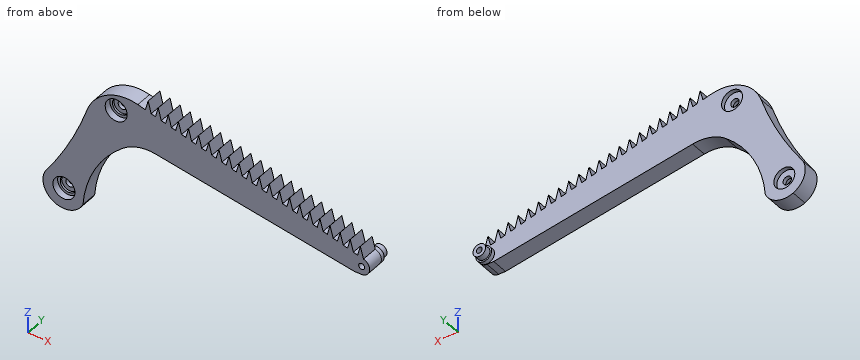
from build123d import *

# Parameters (mm, degrees)
SKETCH1_R                = 1.4
BOSS_EXTRUDE1_DEPTH      = 8
SKETCH2_R                = 3.75
BOSS_EXTRUDE2_DEPTH      = 2
SKETCH3_R                = 3
BOSS_EXTRUDE3_DEPTH      = 3
CUT_EXTRUDE1_DEPTH       = 153.777621068
CUT_EXTRUDE1_DEPTH_BACK  = 153.777621068
SKETCH4_R                = 1.4
FILLET1_R                = 4
SKETCH5_R                = 5.1
CUT_EXTRUDE2_DEPTH       = 3.2
SKETCH6_R                = 4
CUT_EXTRUDE3_DEPTH       = 1
SKETCH7_R                = 5
CUT_EXTRUDE4_DEPTH       = 2
CUT_EXTRUDE5_DEPTH       = 128.709870942
CUT_EXTRUDE5_DEPTH_BACK  = 128.709870942
SKETCH8_R                = 2
SKETCH9_W                = 150
SKETCH9_H                = 50
CUT_EXTRUDE6_DEPTH       = 128.657240829
BOSS_EXTRUDE4_DEPTH      = 8
FILLET2_R                = 10
SKETCH11_R               = 5.25
CUT_EXTRUDE7_DEPTH       = 3.2
SKETCH12_R               = 4
CUT_EXTRUDE8_DEPTH       = 1
SKETCH13_R               = 5
CUT_EXTRUDE9_DEPTH       = 2
CUT_EXTRUDE10_DEPTH      = 128.709870942
CUT_EXTRUDE10_DEPTH_BACK = 128.709870942
SKETCH14_R               = 2
CUT_EXTRUDE11_DEPTH      = 128.657240829
CUT_EXTRUDE11_DEPTH_BACK = 128.657240829
FILLET3_R                = 20
CUT_EXTRUDE12_DEPTH      = 128.657240829
CUT_EXTRUDE12_DEPTH_BACK = 128.657240829
FILLET4_R                = 20
FILLET5_R                = 20
BOSS_EXTRUDE5_DEPTH      = 8
LPATTERN1_COUNT          = 22
LPATTERN1_PITCH          = 5
SKETCH19_R               = 5.25
CUT_EXTRUDE13_DEPTH      = 3.2
SKETCH20_R               = 4
CUT_EXTRUDE14_DEPTH      = 1
CUT_EXTRUDE15_DEPTH      = 129.03726605
CUT_EXTRUDE15_DEPTH_BACK = 129.03726605
SKETCH21_R               = 2
SKETCH22_R               = 5
CUT_EXTRUDE16_DEPTH      = 2


# Some blends are built 0.0001 mm under size
with BuildPart() as part:
    # Sketch1 → Boss-Extrude1 (new body)
    with BuildSketch(Plane(origin=(0, 0, 0), x_dir=(1, 0, 0), z_dir=(0, 1, 0))):
        Polygon((-146.874100845, 0), (146.874100845, 0), (0, -40), align=None)
        with Locations(Location((-117.130755004, -3.915785767, 0), (0, 0, 270))):
            Circle(SKETCH1_R, mode=Mode.SUBTRACT)
        with Locations(Location((0, -30, 0), (0, 0, 270))):
            Circle(SKETCH1_R, mode=Mode.SUBTRACT)
        with Locations(Location((117.130755004, -3.915785767, 0), (0, 0, 270))):
            Circle(SKETCH1_R, mode=Mode.SUBTRACT)
    extrude(amount=BOSS_EXTRUDE1_DEPTH)

    # Sketch2 → Boss-Extrude2 (add)
    with BuildSketch(Plane(origin=(0, 8, 0), x_dir=(1, 0, 0), z_dir=(0, 1, 0))):
        with Locations(Location((117.130755004, -3.915785767, 0), (0, 0, 90))):
            Circle(SKETCH2_R)
    extrude(amount=BOSS_EXTRUDE2_DEPTH)

    # Sketch3 → Boss-Extrude3 (add)
    with BuildSketch(Plane(origin=(0, 10, 0), x_dir=(1, 0, 0), z_dir=(0, 1, 0))):
        with Locations(Location((117.130755004, -3.915785767, 0), (0, 0, 270))):
            Circle(SKETCH3_R)
    extrude(amount=BOSS_EXTRUDE3_DEPTH)

    # Sketch4 → Cut-Extrude1 (cut, two sides: drawn at the far end of the back side and taken through both)
    with BuildSketch(Plane(origin=(0, 13, 0), x_dir=(1, 0, 0), z_dir=(0, 1, 0)).offset(-CUT_EXTRUDE1_DEPTH_BACK)):
        with Locations(Location((117.130755004, -3.915785767, 0), (0, 0, 270))):
            Circle(SKETCH4_R)
    extrude(amount=CUT_EXTRUDE1_DEPTH + CUT_EXTRUDE1_DEPTH_BACK, mode=Mode.SUBTRACT)

    # Fillet1
    fillet1_edges = [part.edges().sort_by_distance(p)[0] for p in [
        (-146.874100845, 4, 0),
        (146.874100845, 4, 0),
    ]]
    fillet(fillet1_edges, radius=FILLET1_R)

    # Sketch5 → Cut-Extrude2 (cut)
    with BuildSketch(Plane.XZ):
        with Locations((-117.130755004, 3.915785767)):
            Circle(SKETCH5_R)
    extrude(amount=-CUT_EXTRUDE2_DEPTH, mode=Mode.SUBTRACT)

    # Sketch6 → Cut-Extrude3 (cut)
    with BuildSketch(Plane.XZ.offset(-3.2)):
        with Locations((-117.130755004, 3.915785767)):
            Circle(SKETCH6_R)
    extrude(amount=-CUT_EXTRUDE3_DEPTH, mode=Mode.SUBTRACT)

    # Sketch7 → Cut-Extrude4 (cut)
    with BuildSketch(Plane(origin=(0, 8, 0), x_dir=(1, 0, 0), z_dir=(0, 1, 0))):
        with Locations((-117.130755004, -3.915785767)):
            Circle(SKETCH7_R)
    extrude(amount=-CUT_EXTRUDE4_DEPTH, mode=Mode.SUBTRACT)

    # Sketch8 → Cut-Extrude5 (cut, two sides: drawn at the far end of the back side and taken through both)
    with BuildSketch(Plane.XZ.offset(-4.2).offset(-CUT_EXTRUDE5_DEPTH_BACK)):
        with Locations(Location((-117.130755004, 3.915785767, 0), (0, 0, 270))):
            Circle(SKETCH8_R)
    extrude(amount=CUT_EXTRUDE5_DEPTH + CUT_EXTRUDE5_DEPTH_BACK, mode=Mode.SUBTRACT)

    # Sketch9 → Cut-Extrude6 (cut, through all)
    with BuildSketch(Plane(origin=(0, 8, 0), x_dir=(1, 0, 0), z_dir=(0, 1, 0))):
        with Locations((-85, -25)):
            Rectangle(SKETCH9_W, SKETCH9_H)
    extrude(amount=-CUT_EXTRUDE6_DEPTH, mode=Mode.SUBTRACT)

    # Sketch10 → Boss-Extrude4 (add)
    with BuildSketch(Plane(origin=(0, 8, 0), x_dir=(1, 0, 0), z_dir=(0, 1, 0))):
        Polygon((-10, -37.276579072), (-38.232590814, 23.268407311), (-20.106435073, 31.720772546), (-5.314795912, 0), (-10, 0), align=None)
    extrude(amount=-BOSS_EXTRUDE4_DEPTH)

    # Fillet2
    fillet2_edges = [part.edges().sort_by_distance(p)[0] for p in [
        (-20.106435073, 4, -31.720772546),
        (-38.232590814, 4, -23.268407311),
    ]]
    fillet(fillet2_edges, radius=FILLET2_R - 0.0001)  # a hair under: the kernel refuses the full size

    # Sketch11 → Cut-Extrude7 (cut)
    with BuildSketch(Plane.XZ):
        with Locations(Location((-24.943330326, -18.431512059, 0), (0, 0, 270))):
            Circle(SKETCH11_R)
    extrude(amount=-CUT_EXTRUDE7_DEPTH, mode=Mode.SUBTRACT)

    # Sketch12 → Cut-Extrude8 (cut)
    with BuildSketch(Plane.XZ.offset(-3.2)):
        with Locations(Location((-24.943330326, -18.431512059, 0), (0, 0, 270))):
            Circle(SKETCH12_R)
    extrude(amount=-CUT_EXTRUDE8_DEPTH, mode=Mode.SUBTRACT)

    # Sketch13 → Cut-Extrude9 (cut)
    with BuildSketch(Plane(origin=(0, 8, 0), x_dir=(1, 0, 0), z_dir=(0, 1, 0))):
        with Locations(Location((-24.943330326, 18.431512059, 0), (0, 0, 270))):
            Circle(SKETCH13_R)
    extrude(amount=-CUT_EXTRUDE9_DEPTH, mode=Mode.SUBTRACT)

    # Sketch14 → Cut-Extrude10 (cut, two sides: drawn at the far end of the back side and taken through both)
    with BuildSketch(Plane.XZ.offset(-4.2).offset(-CUT_EXTRUDE10_DEPTH_BACK)):
        with Locations(Location((-24.943330326, -18.431512059, 0), (0, 0, 270))):
            Circle(SKETCH14_R)
    extrude(amount=CUT_EXTRUDE10_DEPTH + CUT_EXTRUDE10_DEPTH_BACK, mode=Mode.SUBTRACT)

    # Sketch16 → Cut-Extrude11 (cut, two sides: drawn at the far end of the back side and taken through both)
    with BuildSketch(Plane(origin=(0, 8, 0), x_dir=(1, 0, 0), z_dir=(0, 1, 0)).offset(-CUT_EXTRUDE11_DEPTH_BACK)):
        Polygon((-5.314795912, 0), (3.729692447, -19.395967878), (113.729692447, 0), align=None)
    extrude(amount=CUT_EXTRUDE11_DEPTH + CUT_EXTRUDE11_DEPTH_BACK, mode=Mode.SUBTRACT)

    # Fillet3
    fillet3_edges = [part.edges().sort_by_distance(p)[0] for p in [
        (3.729692447, 4, 19.395967878),
    ]]
    fillet(fillet3_edges, radius=FILLET3_R)

    # Sketch17 → Cut-Extrude12 (cut, two sides: drawn at the far end of the back side and taken through both)
    with BuildSketch(Plane(origin=(0, 8, 0), x_dir=(1, 0, 0), z_dir=(0, 1, 0)).offset(-CUT_EXTRUDE12_DEPTH_BACK)):
        with BuildLine():
            Line((-34.006408196, 14.205329441), (-10, -37.276579072))
            ThreePointArc((-10, -37.276579072), (-19.543978786, -10.388869219), (-34.006408196, 14.205329441))
        make_face()
        with BuildLine():
            Line((-15.880252455, 22.657694676), (2.969031552, -12.726090006))
            ThreePointArc((2.969031552, -12.726090006), (-10.157316426, 2.993867794), (-15.880252455, 22.657694676))
        make_face()
    extrude(amount=CUT_EXTRUDE12_DEPTH + CUT_EXTRUDE12_DEPTH_BACK, mode=Mode.SUBTRACT)

    # Fillet4
    # the kernel refuses this fillet: 20 mm, written as the material it takes off along each edge
    with BuildSketch(Plane(origin=(-10, -26.307947418, 37.276579072), x_dir=(-0.2772397367749404, 0, -0.9608007745380734), z_dir=(0, 1, 0))) as fillet4_piece_1:
        with BuildLine():
            CenterArc((11.224724232, -19.987692069), FILLET4_R, 92.010191512, 54.159422267)
            Line((-5.389062305, -8.852967244), (-5.721338035, -8.630272748))
            ThreePointArc((-5.721338035, -8.630272748), (-3.036205438, -4.218496406), (-0.341674286, 0.207987217))
            Line((-0.341674286, 0.207987217), (0.014030905, 0.399753841))
            ThreePointArc((0.014030905, 0.399753841), (5.261589484, 0.307690517), (10.509148062, 0.399753841))
            Line((10.509148062, 0.399753841), (10.523178967, 0))
        make_face()
    extrude(amount=60.615894837, mode=Mode.SUBTRACT)

    # Fillet5
    # the kernel refuses this fillet: 20 mm, written as the material it takes off along each edge
    with BuildSketch(Plane(origin=(0, -51.987814503, 40), x_dir=(-0.6649550163020994, 0, -0.746883408769183), z_dir=(0, 1, 0))) as fillet5_piece_1:
        with BuildLine():
            CenterArc((13.146071877, -18.479501456), FILLET5_R, 67.51430871, 86.041392207)
            Line((-4.761282448, -9.572949875), (-6.552017881, -8.682294717))
            Line((-6.552017881, -8.682294717), (-1.790735433, 0.890655158))
            Line((-1.790735433, 0.890655158), (-1.017670329, 1.721727941))
            ThreePointArc((-1.017670329, 1.721727941), (18.974933836, 2.946825813), (21.560031193, 1.847950146))
            Line((21.560031193, 1.847950146), (20.795125801, 0))
        make_face()
    extrude(amount=111.975629005, mode=Mode.SUBTRACT)

    # Sketch18 → Boss-Extrude5 (add)
    with BuildSketch(Plane(origin=(0, 8, 0), x_dir=(1, 0, 0), z_dir=(0, 1, 0))):
        Polygon((118.015424178, -7.859432398), (116.543976131, -13.442278803), (115.230118761, -8.617988305), align=None)
    boss_extrude5 = extrude(amount=-BOSS_EXTRUDE5_DEPTH)

    # LPattern1: Boss-Extrude5 ×22
    with Locations(*[Vector(-0.9648580996210196, 0, 0.26277147409053875) * (i * LPATTERN1_PITCH) for i in range(1, LPATTERN1_COUNT)]):
        add(boss_extrude5)

    # Sketch19 → Cut-Extrude13 (cut)
    with BuildSketch(Plane.XZ):
        with Locations(Location((0, 30, 0), (0, 0, 270))):
            Circle(SKETCH19_R)
    extrude(amount=-CUT_EXTRUDE13_DEPTH, mode=Mode.SUBTRACT)

    # Sketch20 → Cut-Extrude14 (cut)
    with BuildSketch(Plane.XZ.offset(-3.2)):
        with Locations(Location((0, 30, 0), (0, 0, 270))):
            Circle(SKETCH20_R)
    extrude(amount=-CUT_EXTRUDE14_DEPTH, mode=Mode.SUBTRACT)

    # Sketch21 → Cut-Extrude15 (cut, two sides: drawn at the far end of the back side and taken through both)
    with BuildSketch(Plane.XZ.offset(-4.2).offset(-CUT_EXTRUDE15_DEPTH_BACK)):
        with Locations(Location((0, 30, 0), (0, 0, 270))):
            Circle(SKETCH21_R)
    extrude(amount=CUT_EXTRUDE15_DEPTH + CUT_EXTRUDE15_DEPTH_BACK, mode=Mode.SUBTRACT)

    # Sketch22 → Cut-Extrude16 (cut)
    with BuildSketch(Plane(origin=(0, 8, 0), x_dir=(1, 0, 0), z_dir=(0, 1, 0))):
        with Locations(Location((0, -30, 0), (0, 0, 270))):
            Circle(SKETCH22_R)
    extrude(amount=-CUT_EXTRUDE16_DEPTH, mode=Mode.SUBTRACT)


solid = part.part
Can you work these out from the model? Positions are in its coordinate system, mm. Round coordinates to 2 decimals unless told otherwise and drop trailing zeros. Order: outer loops, then holes, each group sorted by start corner. A loop starts at its lowest first (then second) coordinate and runs counter-clockwise, first axis right, second up. Notation, with made-up numbers: M 25.5,44 L 59.5,44 A17 ccw 59.5,74 Z; hole C -15,78 d2. An arc over 180 degrees is marked long. Use a Markdown table: item, result.
1) If I drill on line 1 along Y through (x, z) = (57, 14); line 2 along X through (y, z) = (6.25, 38.5); line 3 along X through (y, z) = (1.25, -15.5), over which ranges is the centre line in solid material (lowest first)?
Geometry says:
| item | result |
|---|---|
| line 1 | y = 0 to 8 |
| line 2 | x = 14.54 to 15.9, 19.73 to 20.38 |
| line 3 | x = -34.5 to -29.3, -20.59 to -14.8 |
2) I'm going to push flat-ended pins straight in: P1, Ø3, axis at x = -2, z = 30, coming from the +Y side; P2, Ø11.5, axis at x = -1.5, z = 27.5, coming from the -Y side; P3, Ø2, axis at y = 4.5, z = -3, coming from the -X side; P4, Ø6, axis at x = 49, y = 3, coming from the -Z side. Where does each tip first touch, or does it pass through?
Geometry says:
| item | result |
|---|---|
| P1 | stops at y = 6 |
| P2 | stops at y = 0 |
| P3 | stops at x = -27.23 |
| P4 | stops at z = 10.88 |
3) Imagine slicing it at A-A (x = 0). List the corners of the cut face in (y, z) for me.
Geometry says:
| item | result |
|---|---|
| outline | M 0,10.18 L 8,10.18 L 8,25 L 6,25 L 6,28 L 4.2,28 L 4.2,26 L 3.2,26 L 3.2,24.75 L 0,24.75 Z; M 0,35.25 L 3.2,35.25 L 3.2,34 L 4.2,34 L 4.2,32 L 6,32 L 6,35 L 8,35 L 8,37.24 L 0,37.24 Z |
